Here's how the part is built. I have some questions about the finished solid (model axes, mm). Face numbers are marked on the shaded views. A direction names the side the tool comes from. Round coordinates to 2 decimals unless told otherwise and drop trailing zeros. Write each loop counter-clockwise with the first axis right and the second up, starting at its lowest first coordinate (ties: lowest second). Pieces come first, ordered by that corner, then holes. Notation, with made-up numbers: (71.5, 27.25) -> (125.5, 27.25) arc R33 ccw to (125.5, 56.25) -> close; hole circle Ø7 at (23.5, 39). An arc over 180 degrees is marked (long way). Put each result on its own line as item: value. Start each with the question number.
1) I want a section at D-D, the plane x = -32.5. List the corners of the cut face in (y, z) for me.
2) We'd pull the mould along X, two halves only. Please class the marked faces 1, 2 and 3: released by +X, released by -X, zero draft, split by the parting line, or undercut.
3) If I drill on line 1 along Y through (x, z) = (0, 15); line 2 along Y through (x, z) = (0, 6.25); line 3 along X through (y, z) = (-6, 7), over which ranges is the centre line in solid material (lowest first)? Write a range as [from, to].
4) Will these pins go through, and if not, where does the flat tip stop? P1, Ø4, axis at x = 0, y = -32.5, coming from the +Z side; P2, Ø5, axis at x = 4, z = 19, coming from the +Y side; P3, Ø4.5, axis at x = -32.5, y = 0, coming from the -Z side; P4, Ø12, axis at x = -10.5, z = 19.5, coming from the -Y side.
5) Which directions (+Z, -Z, +X, -X, +Y, -Y) give clear straight access to the entire face, cutting with the end or side of a thin tool? Please do the marked faces 4 and 5.
6) I want a section at A-A, the plane x = 0. List the corners of the cut face in (y, z) for me.
7) I want a section at B-B, the plane y = 0. List the corners of the cut face in (x, z) for me, then the cut area to 4 significant figures.
8) I want a section at C-C, the plane z = 21.5. List the corners of the cut face in (x, y) for me.
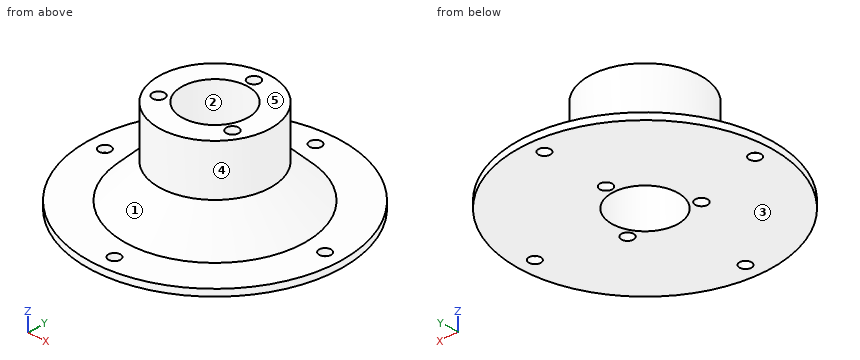
from build123d import *

# Parameters (mm, degrees)
SKETCH_1_R          = 37.5
EXTRUDE_1_DEPTH     = 2
SKETCH_2_R          = 1.75
CUT_EXTRUDE_1_DEPTH = 2
SKETCH_3_R          = 16.5
EXTRUDE_2_DEPTH     = 25
SKETCH_4_R          = 9.75
SKETCH_4_R_2        = 1.8
CUT_EXTRUDE_2_DEPTH = 27
CHAMFER_1_SIZE      = 10


with BuildPart() as part:
    # Эскиз1 → Бобышка-Вытянуть1 (new body)
    with BuildSketch(Plane.XY):
        Circle(SKETCH_1_R)
    extrude(amount=EXTRUDE_1_DEPTH)

    # Эскиз2 → Вырез-Вытянуть1 (cut)
    with BuildSketch(Plane.XY.offset(2)):
        with Locations((0, 32.5)):
            Circle(SKETCH_2_R)
        with Locations((32.5, 0)):
            Circle(SKETCH_2_R)
        with Locations((0, -32.5)):
            Circle(SKETCH_2_R)
        with Locations((-32.5, 0)):
            Circle(SKETCH_2_R)
    extrude(amount=-CUT_EXTRUDE_1_DEPTH, mode=Mode.SUBTRACT)

    # Эскиз3 → Бобышка-Вытянуть2 (add)
    with BuildSketch(Plane.XY.offset(2)):
        Circle(SKETCH_3_R)
    extrude(amount=EXTRUDE_2_DEPTH)

    # Эскиз4 → Вырез-Вытянуть2 (cut)
    with BuildSketch(Plane.XY.offset(27)):
        Circle(SKETCH_4_R)
        with Locations((0, 12.6)):
            Circle(SKETCH_4_R_2)
        with Locations((10.911920088, -6.3)):
            Circle(SKETCH_4_R_2)
        with Locations((-10.911920088, -6.3)):
            Circle(SKETCH_4_R_2)
    extrude(amount=-CUT_EXTRUDE_2_DEPTH, mode=Mode.SUBTRACT)

    # Фаска1
    chamfer_1_edges = [part.edges().sort_by_distance(p)[0] for p in [
        (-16.5, 0, 2),
    ]]
    chamfer(chamfer_1_edges, length=CHAMFER_1_SIZE)


solid = part.part
Findings:
1. outline: (-18.71, 0) -> (-1.75, 0) -> (-1.75, 2) -> (-18.71, 2) -> close; (1.75, 0) -> (18.71, 0) -> (18.71, 2) -> (1.75, 2) -> close
2. face 1: split by the parting line
2. face 2: undercut
2. face 3: zero draft
3. line 1: y = [-16.5, -9.75], [9.75, 10.8], [14.4, 16.5]
3. line 2: y = [-22.25, -9.75], [9.75, 10.8], [14.4, 22.25]
3. line 3: x = [-20.65, -12.69], [-9.14, -7.69], [7.69, 9.14], [12.69, 20.65]
4. P1: stops at z = 2
4. P2: stops at y = 16.43
4. P3: stops at z = 0
4. P4: stops at y = -15.87
5. face 4: +Z
5. face 5: +Z, +X, -X, +Y, -Y
6. outline: (-37.5, 0) -> (-34.25, 0) -> (-34.25, 2) -> (-37.5, 2) -> close; (-30.75, 0) -> (-9.75, 0) -> (-9.75, 27) -> (-16.5, 27) -> (-16.5, 12) -> (-26.5, 2) -> (-30.75, 2) -> close; (9.75, 0) -> (10.8, 0) -> (10.8, 27) -> (9.75, 27) -> close; (14.4, 0) -> (30.75, 0) -> (30.75, 2) -> (26.5, 2) -> (16.5, 12) -> (16.5, 27) -> (14.4, 27) -> close; (34.25, 0) -> (37.5, 0) -> (37.5, 2) -> (34.25, 2) -> close
7. outline: (-37.5, 0) -> (-34.25, 0) -> (-34.25, 2) -> (-37.5, 2) -> close; (-30.75, 0) -> (-9.75, 0) -> (-9.75, 27) -> (-16.5, 27) -> (-16.5, 12) -> (-26.5, 2) -> (-30.75, 2) -> close; (9.75, 0) -> (30.75, 0) -> (30.75, 2) -> (26.5, 2) -> (16.5, 12) -> (16.5, 27) -> (9.75, 27) -> close; (34.25, 0) -> (37.5, 0) -> (37.5, 2) -> (34.25, 2) -> close
7. area: 534.5 mm2
8. outline: circle Ø33 at (0, 0); hole circle Ø3.6 at (-10.91, -6.3); hole circle Ø19.5 at (0, 0); hole circle Ø3.6 at (0, 12.6); hole circle Ø3.6 at (10.91, -6.3)
